from build123d import *

# Parameters (mm, degrees)
SKETCH_1_W                      = 113
SKETCH_1_H                      = 31.5
SKETCH_1_W_2                    = 9.5
SKETCH_1_H_2                    = 11.5
EXTRUDE_1_DEPTH                 = 3
TOOL_D3_R1P5_POWER_CORNERS_R    = 1.5
TOOL_D3_R3_REAR_OUTER_CORNERS_R = 3


with BuildPart() as part:
    # Эскиз1 → Бобышка-Вытянуть1 (new body)
    with BuildSketch(Plane(origin=(0, 0, 0), x_dir=(1, 0, 0), z_dir=(0, 1, 0))):
        with Locations((53.5, -15.75)):
            Rectangle(SKETCH_1_W, SKETCH_1_H)
        with Locations((17.3, -17.3)):
            Rectangle(SKETCH_1_W_2, SKETCH_1_H_2, mode=Mode.SUBTRACT)
    extrude(amount=EXTRUDE_1_DEPTH)

    # tool_D3_R1p5_power_corners
    tool_d3_r1p5_power_corners_edges = [part.edges().sort_by_distance(p)[0] for p in [
        (12.55, 1.5, 11.55),
        (12.55, 1.5, 23.05),
        (22.05, 1.5, 23.05),
        (22.05, 1.5, 11.55),
    ]]
    fillet(tool_d3_r1p5_power_corners_edges, radius=TOOL_D3_R1P5_POWER_CORNERS_R)

    # tool_D3_R3_rear_outer_corners
    tool_d3_r3_rear_outer_corners_edges = [part.edges().sort_by_distance(p)[0] for p in [
        (-3, 3, 15.75),
        (110, 3, 15.75),
    ]]
    fillet(tool_d3_r3_rear_outer_corners_edges, radius=TOOL_D3_R3_REAR_OUTER_CORNERS_R - 0.0001)  # a hair under: the kernel refuses the full size


solid = part.part
The model under review builds one solid part; all positions refer to its coordinate system, in mm. A direction names the side the tool comes from. Round coordinates to 2 decimals unless told otherwise and drop trailing zeros. Order: outer loops, then holes, each group sorted by start corner. A loop starts at its lowest first (then second) coordinate and runs counter-clockwise, first axis right, second up. Notation, with made-up numbers: (16, 16) -> (51, 16) arc R17 ccw to (51, 38) -> close; hole circle Ø10 at (63, 40). An arc over 180 degrees is marked (long way). Write item = value, one per line. Start each with the question number.
Item 1: Clearance check with flat-ended pins moving along their axes: pin 1 Ø1 at (y, z) = (2.5, 12) entering from +X; pin 2 Ø0.9 at (y, z) = (1.5, 17) entering from -X; pin 3 Ø1 at (y, z) = (2, 15.5) entering from +X; pin 4 Ø4 at (x, z) = (40, 14.5) entering from -Y. State where each tip first meets the part, or that it passes through.
Item 2: Mouldability with a two-part tool opening along Z and no side actions: class faces 1 (the face through (53, 0, 16)), 2 (the face through (17, 1, 11.55)), 3 (the face through (53, 1, 31.5)) as released by +Z, released by -Z, zero draft, split by the parting line, or undercut.
Item 3: For faces 4 (the face through (17, 1, 23.05)), 5 (the face through (-2.1, 2.14, 15.53)), list the 3-axis set-ups (+Z, -Z, +X, -X, +Y, -Y) from which the entire face can be reached by the end or side of a thin tool; tool diameter is ignored.
Item 4: For line 1 along X through (y, z) = (0.2, 13.5); line 2 along Z through (x, y) = (20.5, 2.25); line 3 along X through (y, z) = (1.7, 17.5), list the stretches that pass through material, from the lowest coordinate up.
Item 5: Consider section B-B on y = 0.5. Write out the cut boundary in (x, z).
Conclusion:
q1.pin_1 = 109.24
q1.pin_2 = -2.81
q1.pin_3 = 109.6
q1.pin_4 = 0
q2.face_1 = zero draft
q2.face_2 = undercut
q2.face_3 = released by +Z
q3.face_4 = +Y, -Y
q3.face_5 = +Z, -Z, -X, +Y
q4.line_1 = -2.99 to 12.55, 22.05 to 109.99
q4.line_2 = 0 to 11.55, 23.05 to 31.5
q4.line_3 = -2.47 to 12.55, 22.05 to 109.47
q5.outline = (-2.96, 0) -> (109.96, 0) -> (109.96, 31.5) -> (-2.96, 31.5) -> close; hole (12.55, 13.05) arc R1.5 ccw to (14.05, 11.55) -> (20.55, 11.55) arc R1.5 ccw to (22.05, 13.05) -> (22.05, 21.55) arc R1.5 ccw to (20.55, 23.05) -> (14.05, 23.05) arc R1.5 ccw to (12.55, 21.55) -> close
